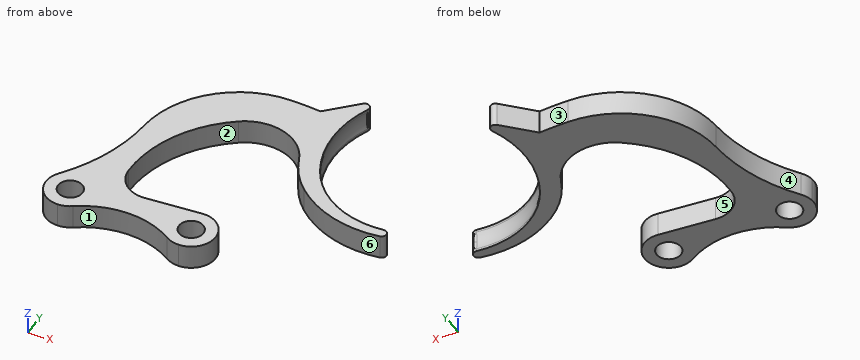
```python
from build123d import *

# Parameters (mm, degrees)
SKETCH_1_R          = 2.5
EXTRUDE_1_DEPTH     = 2.5
SKETCH_2_OUTSIDE_W  = 86.761
SKETCH_2_OUTSIDE_H  = 89.395
CUT_EXTRUDE_1_DEPTH = 5
EXTRUDE_3_DEPTH     = 5
SKETCH_9_R          = 6
FILLET_1_R          = 10
CUT_EXTRUDE_2_DEPTH = 10


with BuildPart() as part:
    # 草圖1 → 填料-伸長1 (new body, symmetric)
    with BuildSketch(Plane.XY):
        with BuildLine():
            Line((0, -5), (25, -5))
            ThreePointArc((25, -5), (29.31444757, -2.526963033), (29.360979806, 2.445783133))
            Line((29.360979806, 2.445783133), (15.064071346, 27.938038866))
            Line((15.064071346, 27.938038866), (44.994741867, 27.938038866))
            Line((44.994741867, 27.938038866), (44.994741867, 63.392785695))
            Line((44.994741867, 63.392785695), (-20.763646925, 63.392785695))
            Line((-20.763646925, 63.392785695), (-20.763646925, 27.938038866))
            Line((-20.763646925, 27.938038866), (-1.414273127, 27.938038866))
            Line((-1.414273127, 27.938038866), (-4.9583743, 0.643835616))
            ThreePointArc((-4.9583743, 0.643835616), (-3.756273292, -3.300062266), (0, -5))
        make_face()
        with Locations((25, 0)):
            Circle(SKETCH_1_R, mode=Mode.SUBTRACT)
        Circle(SKETCH_1_R, mode=Mode.SUBTRACT)
    extrude(amount=EXTRUDE_1_DEPTH, both=True)

    # 草圖2 outside → 除料-伸長1 (cut)
    with BuildSketch(Plane.XY.offset(2.5)):
        with Locations((12.1155, 29.1965)):
            Rectangle(SKETCH_2_OUTSIDE_W, SKETCH_2_OUTSIDE_H)
        with BuildLine():
            Line((31.958651871, 36.150509371), (34.562055634, 40.749856019))
            ThreePointArc((34.562055634, 40.749856019), (29.16979084, 41.362709118), (23.748184909, 41.60415823))
            ThreePointArc((23.748184909, 41.60415823), (9.709628086, 36.160280684), (3.287148618, 22.5415936))
            ThreePointArc((3.287148618, 22.5415936), (1.109618969, 12.24710035), (-3.974011943, 3.034341622))
            ThreePointArc((-3.974011943, 3.034341622), (-3.656567639, -3.410207194), (2.750229007, -4.17567245))
            ThreePointArc((2.750229007, -4.17567245), (12.5, -1.253368592), (22.249770993, -4.17567245))
            ThreePointArc((22.249770993, -4.17567245), (29.842584669, -1.244738415), (24.604254755, 4.984313965))
            Line((24.604254755, 4.984313965), (13.210184283, 4.079645991))
            ThreePointArc((13.210184283, 4.079645991), (8.834388462, 5.55019775), (6.86933477, 9.727358931))
            ThreePointArc((6.86933477, 9.727358931), (13.861035744, 28.211579962), (31.958651871, 36.150509371))
        make_face(mode=Mode.SUBTRACT)
    extrude(amount=-CUT_EXTRUDE_1_DEPTH, mode=Mode.SUBTRACT)

    # 草圖6 → 填料-伸長3 (add)
    with BuildSketch(Plane.XY.offset(2.5)):
        with BuildLine():
            Line((29.843670315, 41.306571089), (35.648712263, 46.914150559))
            ThreePointArc((35.648712263, 46.914150559), (36.916127955, 47.014718803), (37.257884128, 45.79011306))
            ThreePointArc((37.257884128, 45.79011306), (35.304038414, 35.87931312), (37.799168171, 26.090758784))
            ThreePointArc((37.799168171, 26.090758784), (45.415881251, 18.337037181), (56.099880608, 16.340371315))
            ThreePointArc((56.099880608, 16.340371315), (57.209900526, 15.486647675), (56.377991211, 14.360186329))
            ThreePointArc((56.377991211, 14.360186329), (46.455950686, 15.010232793), (37.799168171, 19.902018262))
            ThreePointArc((37.799168171, 19.902018262), (32.860967015, 27.300914678), (31.958651871, 36.150509371))
            Line((31.958651871, 36.150509371), (34.562055634, 40.749856019))
            ThreePointArc((34.562055634, 40.749856019), (32.207046263, 41.063668613), (29.843670315, 41.306571089))
        make_face()
    extrude(amount=-EXTRUDE_3_DEPTH)

    # 除料-掃出3: sweep along a path in 草圖16
    with BuildLine(Plane.XY) as sweep_3_path:
        ThreePointArc((56.099880608, 16.340371315), (45.415881251, 18.337037181), (37.799168171, 26.090758784))
        ThreePointArc((37.799168171, 26.090758784), (35.304038414, 35.87931312), (37.257884128, 45.79011306))
    # 草圖9 → 除料-掃出3 (sweep, cut)
    with BuildSketch(Plane(origin=(37.257884128, 45.79011306, 2.5), x_dir=(0.914403512, -0.404803924, 0), z_dir=(0.404803924, 0.914403512, 0))):
        with Locations((5.663169824, 2.5)):
            Circle(SKETCH_9_R)
    sweep(path=sweep_3_path.line, mode=Mode.SUBTRACT)

    # 圓角1
    fillet_1_edges = [part.edges().sort_by_distance(p)[0] for p in [
        (31.958651871, 36.150509371, 0),
    ]]
    fillet(fillet_1_edges, radius=FILLET_1_R)

    # 草圖20 → 除料-伸長2 (cut)
    with BuildSketch(Plane(origin=(57.238055568, 6.903294961, 0), x_dir=(0, 0, 1), z_dir=(-0.992805403, -0.119739017, 0))):
        with BuildLine():
            Line((1.982046302, 9.505464342), (-1.982046302, 9.505464342))
            ThreePointArc((-1.982046302, 9.505464342), (-1.005231579, 9.25344106), (0, 9.168634166))
            ThreePointArc((0, 9.168634166), (1.005231579, 9.25344106), (1.982046302, 9.505464342))
        make_face()
    extrude(amount=-CUT_EXTRUDE_2_DEPTH, mode=Mode.SUBTRACT)


solid = part.part
```
The model under review builds one solid part; all positions refer to its coordinate system, in mm. Face numbers are marked on the shaded views. A direction names the side the tool comes from. Round coordinates to 2 decimals unless told otherwise and drop trailing zeros. Write each loop counter-clockwise with the first axis right and the second up, starting at its lowest first coordinate (ties: lowest second). Pieces come first, ordered by that corner, then holes.
(1) We need section A-A on y = 1.5. Give the boundary of the cut face in (x, z).
(2) We need section B-B on z = 0.9. Give the number of separate pieces and of enclosed holes in the cut face, and give its area (3 significant figures).
(3) Insertion check: pin 1 (1 mm diameter, centred on y = 27.5, z = 1, fed in from -X); pin 2 (6.5 mm diameter, centred on x = 25, y = 0, fed in from -Z); pin 3 (1 mm diameter, centred on y = 29.5, z = -0.5, fed in from -X). Each pin has a flat end and moves straight along its axis. Give the tip position at first contact, or say it passes through.
(4) Wall thickness on L1, parallel to Y at x = 25, z = 1.5; L2, parallel to Y at x = 0, z = -0.5; L3, parallel to X at y = 23.5, z = 0.85: over which ranges is each line inside the solid? List them lowest first.
(5) Mouldability with a two-part tool opening along Y and no side actions: class the marked faces 4, 5 and 6 as +Y half, -Y half, draft (parallel to the pull), parting line (faces both ways), or undercut.
(6) We need section C-C on x = 5. Give the boundary of the cut face in (y, z), and give its area (3 significant figures).
(7) Machinability: for the marked faces 1, 2 and 3, which of the approach directions +Z, -Z, +X, -X, +Y, -Y give a long, thin tool a straight path to every point of the face, cutting with its end or side? Answer none if there is none.
Findings below:
1. outline: (-4.77, -2.5) - (-2, -2.5) - (-2, 2.5) - (-4.77, 2.5) - close; (2, -2.5) - (23, -2.5) - (23, 2.5) - (2, 2.5) - close; (27, -2.5) - (29.77, -2.5) - (29.77, 2.5) - (27, 2.5) - close
2. separate pieces: 1
2. enclosed holes: 2
2. area: 759 mm2
3. pin 1: stops at x = 4.06
3. pin 2: stops at z = -2.5
3. pin 3: stops at x = 4.76
4. L1: y = -5 to -2.5, 2.5 to 5, 33.36 to 41.58
4. L2: y = -5 to -2.5, 2.5 to 9.6
4. L3: x = 3.37 to 10.33, 34.75 to 39.07
5. face 4: +Y half
5. face 5: undercut
5. face 6: -Y half
6. outline: (-2.92, -2.5) - (29.56, -2.5) - (29.56, 2.5) - (-2.92, 2.5) - close
6. area: 162 mm2
7. face 1: +Z, -Z, -Y
7. face 2: +Z, -Z
7. face 3: +Z, -Z, +Y
